Autodesk Inventor part; units mm, degrees
ref_plane "YZ Plane" through (0, 0, 0) normal (1, 0, 0) x (0, 1, 0)
ref_plane "XZ Plane" through (0, 0, 0) normal (0, 1, 0) x (-1, 0, 0)
ref_plane "XY Plane" through (0, 0, 0) normal (0, 0, 1) x (1, 0, 0)
sketch "Sketch1" plane through (0, 0, 0) normal (0, 0, 1) x (1, 0, 0)
  line L0 (-9.2953, -16.1) -> (-18.5907, 0)
  line L1 (-18.5907, 0) -> (-9.2953, 16.1)
  line L2 (-9.2953, 16.1) -> (9.2953, 16.1)
  line L3 (9.2953, 16.1) -> (18.5907, 0)
  line L4 (18.5907, 0) -> (9.2953, -16.1)
  line L5 (9.2953, -16.1) -> (-9.2953, -16.1)
  circle A0 centre (0, 0) radius 75
  dimension "d0" = 32.2
  dimension "d2" = 150
extrude "Extrusion1" add sketch "Sketch1" along normal blind 10
sketch "Sketch2" plane through (0, 0, 0) normal (0, 0, 1) x (1, 0, 0)
  circle A0 centre (0, 0) radius 75
  line L0 (0, 0) -> (0, 75) construction
  line L1 (0, 95) -> (-15.0761, 73.4691) construction
  line L2 (0, 95) -> (-1.7516, 74.9795)
  circle A1 centre (0, 0) radius 75
  arc A2 (0, 95) -> (-33.7647, 66.9697) centre (-3.8144, 65.2435) ccw
  line L3 (0, 75) -> (0, 95) construction
  point P0 (-1.7516, 74.9795)
  point P1 (-33.7647, 66.9697)
  dimension "d5" = 5
  dimension "d8" = 35
  dimension "d14" = 30
  dimension "d15" = 33
  dimension "d16" = 20
extrude "Extrusion2" add sketch "Sketch2" along normal blind 10 contours A0 A2 L2
pattern_circular "Circular Pattern1" count 6 over 360 about axis through (0, 0, -10) along (0, 0, 1) of "Extrusion2"
equation "\"BendReliefDepth\" = 0.5 * Thickness"
properties part number "NVPH-202 shredder cutter blade" material "Steel"
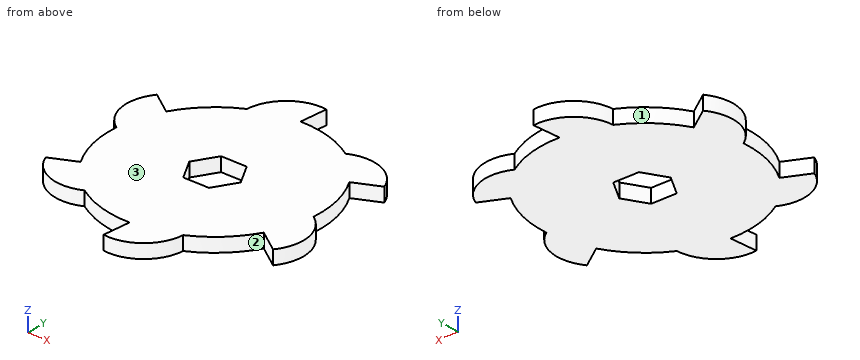
Here's how the part is built. I have some questions about the finished solid (model axes, mm). Face numbers are marked on the shaded views. Round coordinates to 2 decimals unless told otherwise and drop trailing zeros. Loops run counter-clockwise (first coordinate to the right, second up) from the corner with the lowest first, then second, coordinate; pieces in that order, holes last. Notation, with made-up numbers: (-3.5, -5.5) -> (11.5, -5.5) arc R20 ccw to (11.5, 16.5) -> close; hole circle Ø1 at (-37.75, -9). An arc over 180 degrees is marked (long way). Answer as CSV lines item,"result".
1. If we section it at D-D on x = -45: Please give me the cut outline in (y, z), plus the area to 3 significant figures.
Final values:
outline,"(-64.35, 0) -> (60, 0) -> (60, 10) -> (-64.35, 10) -> close"
area,"1,240 mm^2"
2. If we section it at A-A on x = 69: Please give me the cut outline in (y, z).
Final values:
outline,"(-38.21, 0) -> (29.39, 0) -> (29.39, 10) -> (-38.21, 10) -> close; (41.31, 0) -> (62.24, 0) -> (62.24, 10) -> (41.31, 10) -> close"
3. If I drill on L1, parallel to Y at x = 5, z = 7; L2, parallel to Y at x = -3, z = 4; L3, parallel to X at y = -47, z = 3.25, over which ranges is the centre line in solid material (lowest first)?
Final values:
L1,"y = -95.22 to -16.1, 16.1 to 74.83"
L2,"y = -74.94 to -16.1, 16.1 to 95.23"
L3,"x = -81.2 to 58.45, 81.56 to 82.65"
4. For pin 1 (4 mm diameter, centred on x = -45.5, z = 3.5, fed in from +Y); pin 2 (1 mm diameter, centred on y = 37.5, z = 7, fed in from -X); pin 3 (3 mm diameter, centred on x = -0.5, z = 3.5, fed in from +Y); pin 4 (8 mm diameter, centred on x = -1, y = 9.5, fed in from -Z), each with a flat end and sliding along its axis, tell me the tip position at first contact or that it passes through.
Final values:
pin 1,"stops at y = 61.1"
pin 2,"stops at x = -87.41"
pin 3,"stops at y = 95.19"
pin 4,"passes through"
5. Thinking about a two-plate mould opening in X: for the marked faces 1, 2 and 3, which applies, released by +X, released by -X, zero draft, split by the parting line, or undercut?
Final values:
face 1,"undercut"
face 2,"undercut"
face 3,"zero draft"
6. If we section it at B-B on z = 4: Please give me the cut outline in (x, y), plus the area to 3 significant figures.
Final values:
outline,"(-82.27, -47.5) arc R30 ccw to (-41.12, -62.73) arc R75 ccw to (1.75, -74.98) -> (0, -95) arc R30 ccw to (33.76, -66.97) arc R75 ccw to (65.81, -35.97) -> (82.27, -47.5) arc R30 ccw to (74.88, -4.24) arc R75 ccw to (64.06, 39.01) -> (82.27, 47.5) arc R30 ccw to (41.12, 62.73) arc R75 ccw to (-1.75, 74.98) -> (0, 95) arc R30 ccw to (-33.76, 66.97) arc R75 ccw to (-65.81, 35.97) -> (-82.27, 47.5) arc R30 ccw to (-74.88, 4.24) arc R75 ccw to (-64.06, -39.01) -> close; hole (-18.59, 0) -> (-9.3, -16.1) -> (9.3, -16.1) -> (18.59, 0) -> (9.3, 16.1) -> (-9.3, 16.1) -> close"
area,"20,100 mm^2"
7. If we section it at C-C on x = 6.5: Please give me the cut outline in (y, z), plus the area to 3 significant figures.
Final values:
outline,"(-95.12, 0) -> (-16.1, 0) -> (-16.1, 10) -> (-95.12, 10) -> close; (16.1, 0) -> (74.72, 0) -> (74.72, 10) -> (16.1, 10) -> close"
area,"1,380 mm^2"
